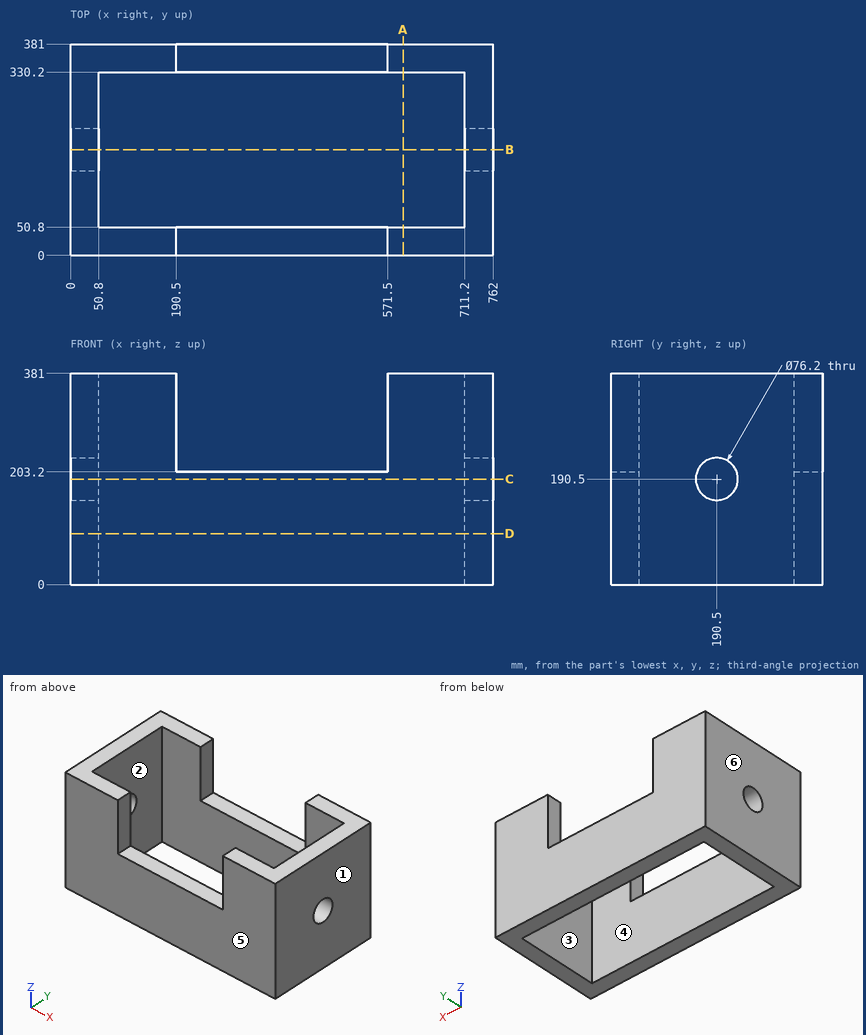
Can you work these out from the drawing? Everything is in mm from the part's minimum corner. A direction names the side the tool comes from. Coordinates: 2 decimals unless noted, no trailing zeros. Loops run counter-clockwise (first coordinate to the right, second up) from the corner with the lowest first, then second, coordinate; pieces in that order, holes last.
1) Imagine slicing it at B-B (y = 190.5). List the corners of the cut face in (x, z) for me, and give its area (3 significant figures).
Reported:
outline: (0, 0) - (50.8, 0) - (50.8, 152.4) - (0, 152.4) - close; (0, 228.6) - (50.8, 228.6) - (50.8, 381) - (0, 381) - close; (711.2, 0) - (762, 0) - (762, 152.4) - (711.2, 152.4) - close; (711.2, 228.6) - (762, 228.6) - (762, 381) - (711.2, 381) - close
area: 31,000 mm2
2) Thinking about a two-plate mould opening in X: for the marked faces 3, 4, 5 and 6, which applies, released by +X, released by -X, zero draft, split by the parting line, or undercut?
Reported:
face 3: undercut
face 4: undercut
face 5: zero draft
face 6: released by -X
3) Imagine slicing it at D-D (z = 92). List the corners of the cut face in (x, y) for me, and give its area (3 significant figures).
Reported:
outline: (0, 0) - (762, 0) - (762, 381) - (0, 381) - close; hole (50.8, 50.8) - (711.2, 50.8) - (711.2, 330.2) - (50.8, 330.2) - close
area: 106,000 mm2
4) Please list where these lines run through material, in increasing order: line 1 along Y through (x, z) = (140.5, 150); line 2 along X through (y, z) = (332.5, 298); line 3 along X through (y, z) = (101, 363.5).
Reported:
line 1: y = 0 to 50.8, 330.2 to 381
line 2: x = 0 to 190.5, 571.5 to 762
line 3: x = 0 to 50.8, 711.2 to 762
5) Imagine slicing it at A-A (x = 599.5). List the corners of the cut face in (y, z) for me.
Reported:
outline: (0, 0) - (50.8, 0) - (50.8, 381) - (0, 381) - close; (330.2, 0) - (381, 0) - (381, 381) - (330.2, 381) - close
6) Which directions (+Z, -Z, +X, -X, +Y, -Y) give clear straight access to the entire face, cutting with the end or side of a thin tool? Please do the marked faces 1 and 2.
Reported:
face 1: +Z, -Z, +X, +Y, -Y
face 2: +Z, -Z
7) Imagine slicing it at C-C (z = 190.5). List the corners of the cut face in (x, y) for me.
Reported:
outline: (0, 0) - (762, 0) - (762, 152.4) - (711.2, 152.4) - (711.2, 50.8) - (50.8, 50.8) - (50.8, 152.4) - (0, 152.4) - close; (0, 228.6) - (50.8, 228.6) - (50.8, 330.2) - (711.2, 330.2) - (711.2, 228.6) - (762, 228.6) - (762, 381) - (0, 381) - close
